Verification items for the finished model (mm, model axes). Face numbers are marked on the shaded views. A direction names the side the tool comes from. Round coordinates to 2 decimals unless told otherwise and drop trailing zeros. Order: outer loops, then holes, each group sorted by start corner. A loop starts at its lowest first (then second) coordinate and runs counter-clockwise, first axis right, second up. Notation, with made-up numbers: (65.5, 53) -> (72.5, 53) arc R13 cw to (72.5, 65) -> close; hole circle Ø2 at (-12, -36.75). An arc over 180 degrees is marked (long way). Write item = value, one per line. Start each with the question number.
from build123d import *

# Parameters (mm, degrees)
FILLET1_R  = 1.3
SKETCH2_W  = 9.3
SKETCH2_H  = 1.2
SLOT_DEPTH = 1.4


with BuildPart() as part:
    # BodySke → Base-Revolve (revolve)
    with BuildSketch(Plane.XY):
        Polygon((0, 0), (0, 4.65), (0.55, 4.65), (2.7, 2.5), (16, 2.5), (16, 0), align=None)
    revolve(axis=Axis((-6.35, 0, 0), (1, 0, 0)))

    # Fillet1
    fillet1_edges = [part.edges().sort_by_distance(p)[0] for p in [
        (2.7, -2.5, 0),
    ]]
    fillet(fillet1_edges, radius=FILLET1_R)

    # Sketch2 → Slot (cut)
    with BuildSketch(Plane.ZY):
        Rectangle(SKETCH2_W, SKETCH2_H)
    extrude(amount=-SLOT_DEPTH, mode=Mode.SUBTRACT)


solid = part.part
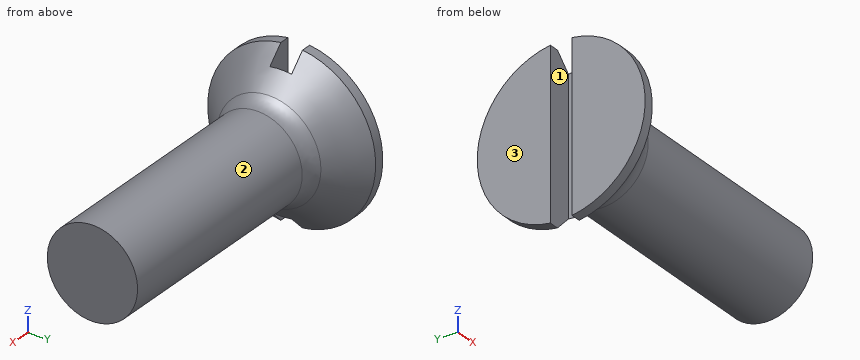
(1) Cross-section at A-A (x = 10). Enter the section's corners in (y, z).
(2) Set-up check for the marked faces 1, 2 and 3: record each of +Z, -Z, +X, -X, +Y, -Y from which the full face is reachable in a straight line by a thin tool's end or side.
(3) Depth check by flat-ended pin: pin 1 (3 mm diameter, centred on x = 12.5, z = -2, fed in from +Y); pin 2 (0.7 mm diameter, centred on x = 0.5, z = 0.5, fed in from +Y); pin 3 (2 mm diameter, centred on x = 6.5, y = 1, fed in from +Z). Enter the tip coordinate at first touch or a pass-through.
(4) Scan lines: line 1 along Z through (x, y) = (13.75, 0); line 2 along X through (y, z) = (4.25, -1.5); line 3 along X through (y, z) = (-2.25, 4). Record each from-to range of solid material in increasing order. Write a range as from..to.
Outcome:
q1.outline = circle Ø5 at (0, 0)
q2.face_1 = +Z, -Z, -X
q2.face_2 = +X
q2.face_3 = +Z, -Z, -X, +Y, -Y
q3.pin_1 = 2.45
q3.pin_2 = 4.65
q3.pin_3 = 2.5
q4.line_1 = -2.5..2.5
q4.line_2 = 0..0.69
q4.line_3 = 0..0.61
